from build123d import *

# Parameters (mm, degrees)
SKETCH1_W           = 21.59
SKETCH1_H           = 63.5
SKETCH1_R           = 4.124999878
SKETCH1_R_2         = 3.5052
BOSS_EXTRUDE1_DEPTH = 3.175
FILLET1_R           = 3.175


with BuildPart() as part:
    # Sketch1 → Boss-Extrude1 (new body)
    with BuildSketch(Plane.XY):
        with Locations((10.795, 31.75)):
            Rectangle(SKETCH1_W, SKETCH1_H)
        with Locations((10.795, 9.525)):
            Circle(SKETCH1_R, mode=Mode.SUBTRACT)
        with Locations(Location((10.795, 57.15, 0), (0, 0, 180))):
            Circle(SKETCH1_R_2, mode=Mode.SUBTRACT)
    extrude(amount=BOSS_EXTRUDE1_DEPTH)

    # Fillet1
    fillet1_edges = [part.edges().sort_by_distance(p)[0] for p in [
        (0, 0, 1.5875),
        (21.59, 0, 1.5875),
        (21.59, 63.5, 1.5875),
        (0, 63.5, 1.5875),
    ]]
    fillet(fillet1_edges, radius=FILLET1_R)


solid = part.part
Could you check a few things on this model? Use its own coordinates, in mm. Coordinates: 2 decimals unless noted, no trailing zeros. Loops run counter-clockwise (first coordinate to the right, second up) from the corner with the lowest first, then second, coordinate; pieces in that order, holes last. Notation, with made-up numbers: (-34.5, 83) -> (-10.5, 83) arc R24 cw to (-10.5, 107) -> close; hole circle Ø11 at (68, 21.25). An arc over 180 degrees is marked (long way). Answer in a Markdown table with one row per item.
(1) If I drill on probe 1 along Y at (x, z) = (11, 2.8); probe 2 along Y at (x, z) = (10.75, 2.9); probe 3 along X at (y, z) = (57.15, 2.5), over which ranges is the centre line in solid material (lowest first)?
Results found:
| item | result |
|---|---|
| probe 1 | y = 0 to 5.41, 13.64 to 53.65, 60.65 to 63.5 |
| probe 2 | y = 0 to 5.4, 13.65 to 53.65, 60.65 to 63.5 |
| probe 3 | x = 0 to 7.29, 14.3 to 21.59 |
(2) Imagine slicing it at A-A (y = 57.15). List the corners of the cut face in (x, z) for me (3 decimals).
Results found:
| item | result |
|---|---|
| outline | (0, 0) -> (7.29, 0) -> (7.29, 3.175) -> (0, 3.175) -> close; (14.3, 0) -> (21.59, 0) -> (21.59, 3.175) -> (14.3, 3.175) -> close |
(3) Imagine slicing it at B-B (z = 1.1). List the corners of the cut face in (x, y) for me (3 decimals), plus the area to 3 significant figures.
Results found:
| item | result |
|---|---|
| outline | (0, 3.175) arc R3.175 ccw to (3.175, 0) -> (18.415, 0) arc R3.175 ccw to (21.59, 3.175) -> (21.59, 60.325) arc R3.175 ccw to (18.415, 63.5) -> (3.175, 63.5) arc R3.175 ccw to (0, 60.325) -> close; hole circle Ø8.25 at (10.795, 9.525); hole circle Ø7.01 at (10.795, 57.15) |
| area | 1,270 mm^2 |
